Input: part model. Units: mm. Frame: model coordinates. Face numbers are marked on the shaded views. Round coordinates to 2 decimals unless told otherwise and drop trailing zeros. Loops run counter-clockwise (first coordinate to the right, second up) from the corner with the lowest first, then second, coordinate; pieces in that order, holes last. Notation, with made-up numbers: M 29,86 L 64,86 A18 ccw 64,113 Z; hole C 0.5,50 d3. An arc over 180 degrees is marked long. Put each result on its own line as item: value. Start each with the question number.
1) Draft query along Y for the marked faces 1, 2 and 3. Return one class per face: +Y half, -Y half, draft (parallel to the pull), parting line (faces both ways), or undercut.
2) Pin query (flat end, axial travel): pin 1 (4 mm diameter, centred on y = 6, z = 10.5, fed in from -X); pin 2 (1 mm diameter, centred on y = -1.5, z = 16, fed in from -X); pin 3 (1.6 mm diameter, centred on x = -340, y = -4, fed in from +Z). Return the tip coordinate at first contact, or that it passes through.
3) Section A-A on z = 10.5. Output: boundary loops of the cut face in (x, y), plus the area to 3 significant figures.
4) Section D-D on y = -4. Output: boundary loops of the cut face in (x, z), plus the area to 3 significant figures.
5) Line query: probe 1 along Y at (x, z) = (-341.5, 17.5); probe 2 along X at (y, z) = (6.75, 10); probe 3 along X at (y, z) = (-5, 7.5). Output: solid intervals per line, ascending.
6) Section B-B on x = -341. Output: boundary loops of the cut face in (y, z).
7) Section C-C on z = 4.5. Output: boundary loops of the cut face in (x, y).
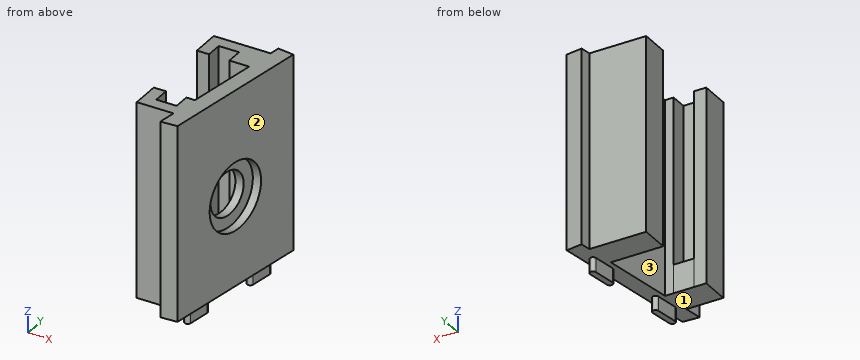
from build123d import *

# Parameters (mm, degrees)
BOSS_EXTRUDE1_DEPTH = 24
BOSS_EXTRUDE2_DEPTH = 1.75
CUT_EXTRUDE1_START  = -20.5
CUT_EXTRUDE1_DEPTH  = 20.5
SKETCH6_R           = 2.7
CUT_EXTRUDE2_DEPTH  = 29.350689779
CUT_EXTRUDE3_REACH  = 30.351
SKETCH7_R           = 4.2


with BuildPart() as part:
    # Sketch1 → Boss-Extrude1 (new body)
    with BuildSketch(Plane.XY):
        Polygon((-343.150061909, -6.552014413), (-338.636620437, -6.533511206), (-338.962584075, -8.694184464), (-336.922787571, -8.580403809), (-334.068528094, 10.339259009), (-336.052092086, 10.598219582), (-336.243956758, 9.326430897), (-343.215039679, 9.297852397), (-343.200758501, 5.814279983), (-341.700745896, 5.814279983), (-341.708902968, 7.804014317), (-339.208923976, 7.814263177), (-339.200724888, 5.814279983), (-336.772305205, 5.82423548), (-338.108271991, -3.031315789), (-339.164443925, -3.035645649), (-339.156244837, -5.035628842), (-341.656223829, -5.045877702), (-341.664422917, -3.045894508), (-343.164410312, -3.052043824), align=None)
        Polygon((-341.708902968, 7.804014317), (-341.700745896, 5.814279983), (-339.200724888, 5.814279983), (-339.208923976, 7.814263177), align=None)
        Polygon((-341.664422917, -3.045894508), (-339.164443925, -3.035645649), (-339.156244837, -5.035628842), (-341.656223829, -5.045877702), align=None)
    extrude(amount=BOSS_EXTRUDE1_DEPTH)

    # Sketch2 → Boss-Extrude2 (add)
    with BuildSketch(Plane(origin=(0, 0, 0), x_dir=(-1, 0, 0), z_dir=(0, 0, -1))):
        with BuildLine():
            Line((335.897375602, 7.434032542), (336.307604283, 4.714802425))
            ThreePointArc((336.307604283, 4.714802425), (335.992740451, 4.288058043), (335.565996069, 4.602921876))
            Line((335.565996069, 4.602921876), (335.155767388, 7.322151993))
            ThreePointArc((335.155767388, 7.322151993), (335.47063122, 7.748896374), (335.897375602, 7.434032542))
        make_face()
        with BuildLine():
            Line((337.437092292, -2.772089521), (337.847320974, -5.491319638))
            ThreePointArc((337.847320974, -5.491319638), (337.532457142, -5.918064019), (337.10571276, -5.603200187))
            Line((337.10571276, -5.603200187), (336.695484079, -2.88397007))
            ThreePointArc((336.695484079, -2.88397007), (337.010347911, -2.457225689), (337.437092292, -2.772089521))
        make_face()
    extrude(amount=BOSS_EXTRUDE2_DEPTH)

    # Sketch3 → Cut-Extrude1 (cut)
    with BuildSketch(Plane.XY.offset(24).offset(CUT_EXTRUDE1_START)):
        Polygon((-339.156244837, -5.035628842), (-341.656223829, -5.045877702), (-341.664422917, -3.045894508), (-339.164443925, -3.035645649), align=None)
        Polygon((-341.708902968, 7.804014317), (-341.700745896, 5.814279983), (-339.200724888, 5.814279983), (-339.208923976, 7.814263177), align=None)
    extrude(amount=CUT_EXTRUDE1_DEPTH, mode=Mode.SUBTRACT)

    # Sketch6 → Cut-Extrude2 (cut, through all)
    with BuildSketch(Plane(origin=(-334.020527762, -1.369343309, 0), x_dir=(0, 0, -1), z_dir=(-0.9999915968347833, -0.00409954385515742, 0))):
        with Locations(Location((-11, -2.254799372, 0), (0, 0, 270))):
            Circle(SKETCH6_R)
    extrude(amount=CUT_EXTRUDE2_DEPTH, mode=Mode.SUBTRACT)

    # Cut-Extrude3: up to this plane
    cut_extrude3_end = Plane(origin=(-329.148436726, 49.656014161, 45.350773476), z_dir=(-0.9888109516181178, 0.14917406597687244, 0))
    # Sketch7 → Cut-Extrude3 (cut, up to the surface)
    with BuildSketch(Plane(origin=(-334.020527762, -1.369343309, 0), x_dir=(0, 0, -1), z_dir=(-0.9999915968347833, -0.00409954385515742, 0)), mode=Mode.PRIVATE) as cut_extrude3_sk1:
        with Locations(Location((-11, -2.254799372, 0), (0, 0, 270))):
            Circle(SKETCH7_R)
    cut_extrude3_tool1 = split(extrude(cut_extrude3_sk1.sketch, amount=CUT_EXTRUDE3_REACH, mode=Mode.PRIVATE), bisect_by=cut_extrude3_end, keep=Keep.BOTH, mode=Mode.PRIVATE)
    add(cut_extrude3_tool1.solids().sort_by_distance((-334.029771, 0.885437, 11))[0], mode=Mode.SUBTRACT)


solid = part.part
Geometry results:
1. face 1: draft
1. face 2: -Y half
1. face 3: undercut
2. pin 1: stops at x = -343.21
2. pin 2: stops at x = -337.95
2. pin 3: stops at z = 3.5
3. outline: M -343.22,9.3 L -343.2,5.81 L -341.7,5.81 L -341.71,7.8 L -339.21,7.81 L -339.2,5.81 L -336.77,5.82 L -337.12,3.53 L -336.11,3.53 L -335.88,5.05 L -334.87,5.05 L -334.07,10.34 L -336.05,10.6 L -336.24,9.33 Z; M -343.16,-3.05 L -343.15,-6.55 L -338.64,-6.53 L -338.96,-8.69 L -336.92,-8.58 L -336.13,-3.29 L -337.14,-3.3 L -336.91,-1.78 L -337.92,-1.78 L -338.11,-3.03 L -339.16,-3.04 L -339.16,-5.04 L -341.66,-5.05 L -341.66,-3.05 Z
3. area: 55.0 mm²
4. outline: M -343.16,0 L -337.62,0 L -337.62,-1.75 L -336.86,-1.75 L -336.86,0 L -336.23,0 L -336.23,24 L -339.16,24 L -339.16,3.5 L -341.66,3.5 L -341.66,24 L -343.16,24 Z
4. area: 116 mm²
5. probe 1: y = -6.55 to -5.05, 7.8 to 9.3
5. probe 2: x = -343.2 to -341.7, -339.2 to -334.61
5. probe 3: x = -343.16 to -341.66, -339.16 to -336.38
6. outline: M -6.54,0 L -3.04,0 L -3.04,3.5 L -5.04,3.5 L -5.04,24 L -6.54,24 Z; M 5.81,0 L 9.31,0 L 9.31,24 L 7.81,24 L 7.81,3.5 L 5.81,3.5 Z
7. outline: M -343.22,9.3 L -343.2,5.81 L -341.7,5.81 L -341.71,7.8 L -339.21,7.81 L -339.2,5.81 L -336.77,5.82 L -338.11,-3.03 L -339.16,-3.04 L -339.16,-5.04 L -341.66,-5.05 L -341.66,-3.05 L -343.16,-3.05 L -343.15,-6.55 L -338.64,-6.53 L -338.96,-8.69 L -336.92,-8.58 L -334.07,10.34 L -336.05,10.6 L -336.24,9.33 Z
